Here's the drawing with two shaded views (mm, measured from the low corner). I have some questions. Give positions to 0.01 mm unless a question says otherwise; leave off trailing zeros. Loops run counter-clockwise (first coordinate to the right, second up) from the corner with the lowest first, then second, coordinate; pieces in that order, holes last. Notation, with made-up numbers: (54.25, -19.5) - (90.25, -19.5) arc R20 cw to (90.25, 16.5) - close; hole circle Ø11 at (55.5, 67.25). An arc over 180 degrees is marked (long way). Answer as a JSON object with one key per item and string values. Group by question number.
Item 1: Suppose I cut it at B-B on z = 10.5. Write out the boundary of the cut face in (x, y).
Item 2: Suppose I cut it at C-C on y = 19.5. Write out the boundary of the cut face in (x, z).
Item 3: Please list where these lines run through material, in increasing order: L1, parallel to Z at x = 19.5, y = 59; L2, parallel to Y at x = 18, z = 13.
Item 4: Suppose I cut it at A-A on x = 11.5. Write out the boundary of the cut face in (y, z).
Item 5: Thinking about a two-plate mould opening in Y: for the marked faces 1, 2 and 3, which applies, pulls with the +Y half, pulls with the -Y half, needs draft (parallel to the pull), parting line crosses it, or undercut?
Item 6: Will these pins go through, and if not, where does the flat tip stop? pin 1 (6 mm diameter, centred on x = 13, z = 24, fed in from -Y); pin 2 (5 mm diameter, centred on x = 9.5, y = 22.5, fed in from +Z).
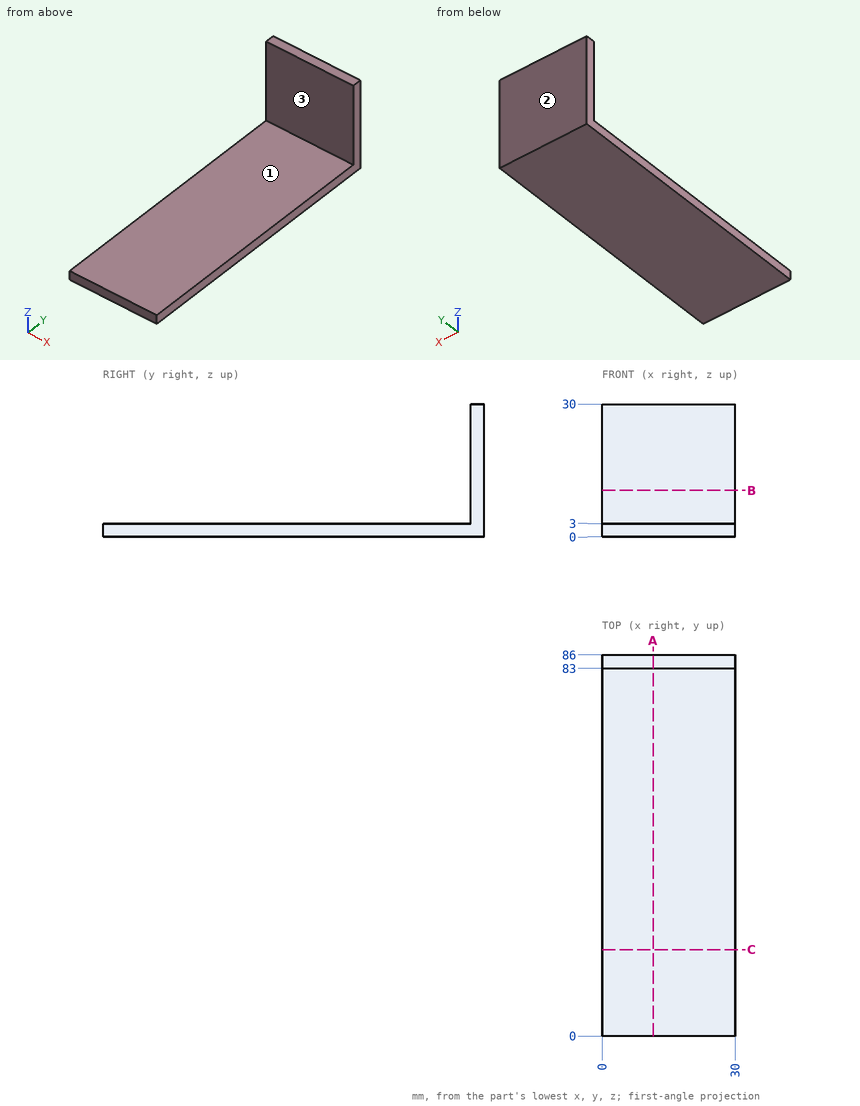
Worked out:
{
 "1": {"outline": "(0, 83) - (30, 83) - (30, 86) - (0, 86) - close"},
 "2": {"outline": "(0, 0) - (30, 0) - (30, 3) - (0, 3) - close"},
 "3": {"L1": "z = 0 to 3", "L2": "y = 83 to 86"},
 "4": {"outline": "(0, 0) - (86, 0) - (86, 30) - (83, 30) - (83, 3) - (0, 3) - close"},
 "5": {"face 1": "needs draft", "face 2": "pulls with the +Y half", "face 3": "pulls with the -Y half"},
 "6": {"pin 1": "stops at y = 83", "pin 2": "stops at z = 3"}
}
